Build history of the part. All positions in model axes, mm. A direction names the side the tool comes from. Round coordinates to 2 decimals unless told otherwise and drop trailing zeros. Order: outer loops, then holes, each group sorted by start corner. A loop starts at its lowest first (then second) coordinate and runs counter-clockwise, first axis right, second up. Notation, with made-up numbers: (43.25, 70) -> (57.25, 70) arc R19 cw to (57.25, 103) -> close; hole circle Ø5 at (15, 31). An arc over 180 degrees is marked (long way). Use a Markdown table: item, result. Add a question column.
Item 1: Probe L1, parallel to X at y = 0.2, z = -0.8 (3 decimals); L2, parallel to X at y = -0.55, z = -1; L3, parallel to Z at x = -2, y = -0.1. List the from-to ranges inside material, lowest first.
Item 2: Slice it at C-C, the plane x = 2. Give the cut face in (y, z).
Item 3: Slice it at B-B, the plane z = 0. Give the cut face in (x, y) (3 decimals), plus the area to 3 significant figures.
Item 4: 3-axis set-ups, long thin cutter, end or side, ignore diameter. For faces 1 (the face through (-1.421, 0.604, 0.753)), 2 (the face through (0, -1, -1)), 3 (the face through (-1, 1.6, 0.8)): which of +Z, -Z, +X, -X, +Y, -Y reach the whole face in a straight line?
Item 5: Pin check, flat tips, straight feed: pin 1 (1 mm diameter, centred on x = 0, y = -1, fed in from -Z); pin 2 (1.5 mm diameter, centred on x = 1, y = 0.5, fed in from +Z); pin 3 (1.5 mm diameter, centred on x = 3.5, z = 0, fed in from -Y); pin 4 (1.5 mm diameter, centred on x = -1.5, z = -0.5, fed in from -Y). Stop position of each tip, or through.
Item 6: Two-plate mould, pull along Y, no slides. Class faces 4 (the face through (-1.421, -0.604, -0.753)), 5 (the face through (6.35, 0, 0)), 6 (the face through (3.03, -0.33, 1.04)): released by +Y, released by -Y, zero draft, split by the parting line, or undercut.
from build123d import *

# Parameters (mm, degrees)
CHAMFER1_SIZE      = 0.2032
CHAMFER2_SIZE      = 0.127
CUT_EXTRUDE1_DEPTH = 1.5494


with BuildPart() as part:
    # Sketch1 → Revolve1 (revolve)
    with BuildSketch(Plane.XY, mode=Mode.PRIVATE) as revolve1_sk:
        Polygon((-2.1844, 0), (6.35, 0), (6.35, 1.0922), (0, 1.0922), (0, 1.7907), (-2.1844, 1.7907), align=None)
    revolve(revolve1_sk.sketch.rotate(Axis((-2.1844, 0, 0), (1, 0, 0)), 90), axis=Axis((-2.1844, 0, 0), (1, 0, 0)))

    # Chamfer1
    chamfer1_edges = [part.edges().sort_by_distance(p)[0] for p in [
        (6.35, 0, -1.0922),
    ]]
    chamfer(chamfer1_edges, length=CHAMFER1_SIZE)

    # Chamfer2
    chamfer2_edges = [part.edges().sort_by_distance(p)[0] for p in [
        (-2.1844, 0, -1.7907),
    ]]
    chamfer(chamfer2_edges, length=CHAMFER2_SIZE)

    # Sketch2 → Cut-Extrude1 (cut)
    with BuildSketch(Plane.ZY.offset(2.1844)):
        Polygon((1.100183814, 0.178167419), (0.395794396, 1.041870841), (-0.704389418, 0.863703422), (-1.100183814, -0.178167419), (-0.395794396, -1.041870841), (0.704389418, -0.863703422), align=None)
    extrude(amount=-CUT_EXTRUDE1_DEPTH, mode=Mode.SUBTRACT)


solid = part.part
Check sheet entries:
| question | item | result |
|---|---|---|
| 1 | L1 | -0.635 to 6.35 |
| 1 | L2 | -2.18 to 0 |
| 1 | L3 | -1.79 to -1.07, 0.99 to 1.79 |
| 2 | outline | circle Ø2.18 at (0, 0) |
| 3 | outline | (-2.184, -1.664) -> (-2.057, -1.791) -> (0, -1.791) -> (0, -1.092) -> (6.147, -1.092) -> (6.35, -0.889) -> (6.35, 0.889) -> (6.147, 1.092) -> (0, 1.092) -> (0, 1.791) -> (-2.057, 1.791) -> (-2.184, 1.664) -> (-2.184, 0.978) -> (-0.635, 0.978) -> (-0.635, -0.978) -> (-2.184, -0.978) -> close |
| 3 | area | 18.6 mm2 |
| 4 | face 1 | -X |
| 4 | face 2 | +X |
| 4 | face 3 | +X, -X |
| 5 | pin 1 | z = -1.72 |
| 5 | pin 2 | z = 1.09 |
| 5 | pin 3 | y = -1.09 |
| 5 | pin 4 | y = -1.79 |
| 6 | face 4 | undercut |
| 6 | face 5 | zero draft |
| 6 | face 6 | split by the parting line |
